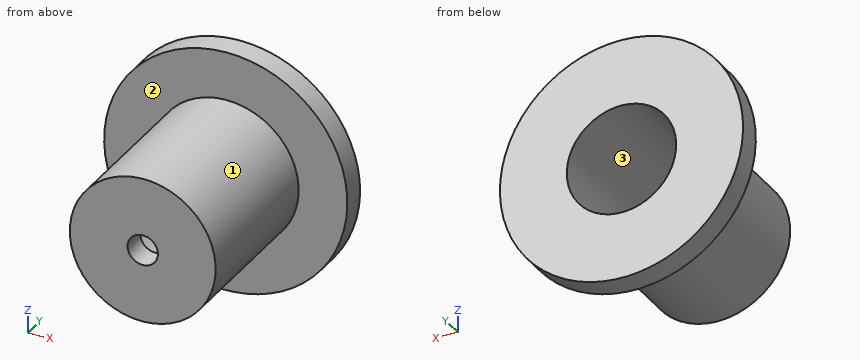
```python
from build123d import *

# Parameters (mm, degrees)
ESQUISSE1_R             = 6
BOSS_EXTRU_1_DEPTH      = 15
ESQUISSE3_R             = 10
BOSS_EXTRU_2_DEPTH      = 2
ESQUISSE2_R             = 4.5
ENL_V_MAT_EXTRU_2_DEPTH = 13
ESQUISSE4_R             = 1.25
ENL_V_MAT_EXTRU_3_DEPTH = 20.209372712


with BuildPart() as part:
    # Esquisse1 → Boss.-Extru.1 (new body)
    with BuildSketch(Plane(origin=(0, 0, 0), x_dir=(1, 0, 0), z_dir=(0, 1, 0))):
        with Locations(Location((0, 0, 0), (0, 0, 270))):
            Circle(ESQUISSE1_R)
    extrude(amount=BOSS_EXTRU_1_DEPTH)

    # Esquisse3 → Boss.-Extru.2 (add)
    with BuildSketch(Plane(origin=(0, 15, 0), x_dir=(1, 0, 0), z_dir=(0, 1, 0))):
        with Locations(Location((0, 0, 0), (0, 0, 270))):
            Circle(ESQUISSE3_R)
    extrude(amount=-BOSS_EXTRU_2_DEPTH)

    # Esquisse2 → Enlèv. mat.-Extru.2 (cut)
    with BuildSketch(Plane(origin=(0, 15, 0), x_dir=(1, 0, 0), z_dir=(0, 1, 0))):
        with Locations(Location((0, 0, 0), (0, 0, 270))):
            Circle(ESQUISSE2_R)
    extrude(amount=-ENL_V_MAT_EXTRU_2_DEPTH, mode=Mode.SUBTRACT)

    # Esquisse4 → Enlèv. mat.-Extru.3 (cut, through all)
    with BuildSketch(Plane(origin=(0, 2, 0), x_dir=(1, 0, 0), z_dir=(0, 1, 0))):
        with Locations(Location((0, 0, 0), (0, 0, 270))):
            Circle(ESQUISSE4_R)
    extrude(amount=-ENL_V_MAT_EXTRU_3_DEPTH, mode=Mode.SUBTRACT)


solid = part.part
```
CAD build for the part. Positions are in the model's coordinates, mm. Face numbers are marked on the shaded views. Round coordinates to 2 decimals unless told otherwise and drop trailing zeros. Loops run counter-clockwise (first coordinate to the right, second up) from the corner with the lowest first, then second, coordinate; pieces in that order, holes last. Notation, with made-up numbers: M -32,26.25 L 12,26.25 A14 cw 12,42.25 Z; hole C 26,32.25 d1. An arc over 180 degrees is marked long. Use a Markdown table: item, result. Add a question column.
(1) Cut at A-A (z = 0). Give the cut face in (x, y), and give its area (3 significant figures).
(2) Flat gauge pins, fed straight in: pin 1 (5 mm diameter, centred on x = 3.5, y = 7.5, fed in from +Z); pin 2 (1.5 mm diameter, centred on x = -5.5, y = 3.5, fed in from +Z); pin 3 (2 mm diameter, centred on y = 7.5, z = 0, fed in from +X). Where does each tip first touch, or does it go through?
(3) Drill centre lines: line 1 (X direction, y = 0.5, z = 0); line 2 (X direction, y = 7, z = 0); line 3 (Y direction, x = -5.5, z = -3.25). Where is each one in solid material? Low to high.
(4) Pull direction Z, two halves, no side cores. Call the marked faces 1, 2 and 3: +Z half, -Z half, draft (parallel to the pull), parting line (faces both ways), or undercut.
(5) Cut at B-B (y = 14.25). Give the cut face in (x, z), and give its area (3 significant figures).
(6) Cut at C-C (z = -3.5). Give the cut face in (x, y).
(7) Cut at D-D (x = 3.25). Give the cut face in (y, z), and give its area (3 significant figures).
Geometry says:
| question | item | result |
|---|---|---|
| 1 | outline | M -10,13 L -6,13 L -6,0 L -1.25,0 L -1.25,2 L -4.5,2 L -4.5,15 L -10,15 Z; M 1.25,0 L 6,0 L 6,13 L 10,13 L 10,15 L 4.5,15 L 4.5,2 L 1.25,2 Z |
| 1 | area | 74.0 mm² |
| 2 | pin 1 | stops at z = 5.92 |
| 2 | pin 2 | stops at z = 3.67 |
| 2 | pin 3 | stops at x = 6 |
| 3 | line 1 | x = -6 to -1.25, 1.25 to 6 |
| 3 | line 2 | x = -6 to -4.5, 4.5 to 6 |
| 3 | line 3 | y = 13 to 15 |
| 4 | face 1 | parting line |
| 4 | face 2 | draft |
| 4 | face 3 | undercut |
| 5 | outline | C 0,0 d20; hole C 0,0 d9 |
| 5 | area | 251 mm² |
| 6 | outline | M -9.37,13 L -4.87,13 L -4.87,0 L 4.87,0 L 4.87,13 L 9.37,13 L 9.37,15 L 2.83,15 L 2.83,2 L -2.83,2 L -2.83,15 L -9.37,15 Z |
| 7 | outline | M 0,-5.04 L 13,-5.04 L 13,-9.46 L 15,-9.46 L 15,-3.11 L 2,-3.11 L 2,3.11 L 15,3.11 L 15,9.46 L 13,9.46 L 13,5.04 L 0,5.04 Z |
| 7 | area | 88.0 mm² |
